Source: three-view drawing plus pictorial views. Frame: mm from the lowest corner of the part. A direction names the side the tool comes from. Round coordinates to 2 decimals unless told otherwise and drop trailing zeros. Loops run counter-clockwise (first coordinate to the right, second up) from the corner with the lowest first, then second, coordinate; pieces in that order, holes last. Notation, with made-up numbers: M 42.5,76.5 L 91.5,76.5 A17 ccw 91.5,98.5 Z; hole C 11,51 d7. An arc over 180 degrees is marked long. Write each question's results on one line, items separated by ' | '.
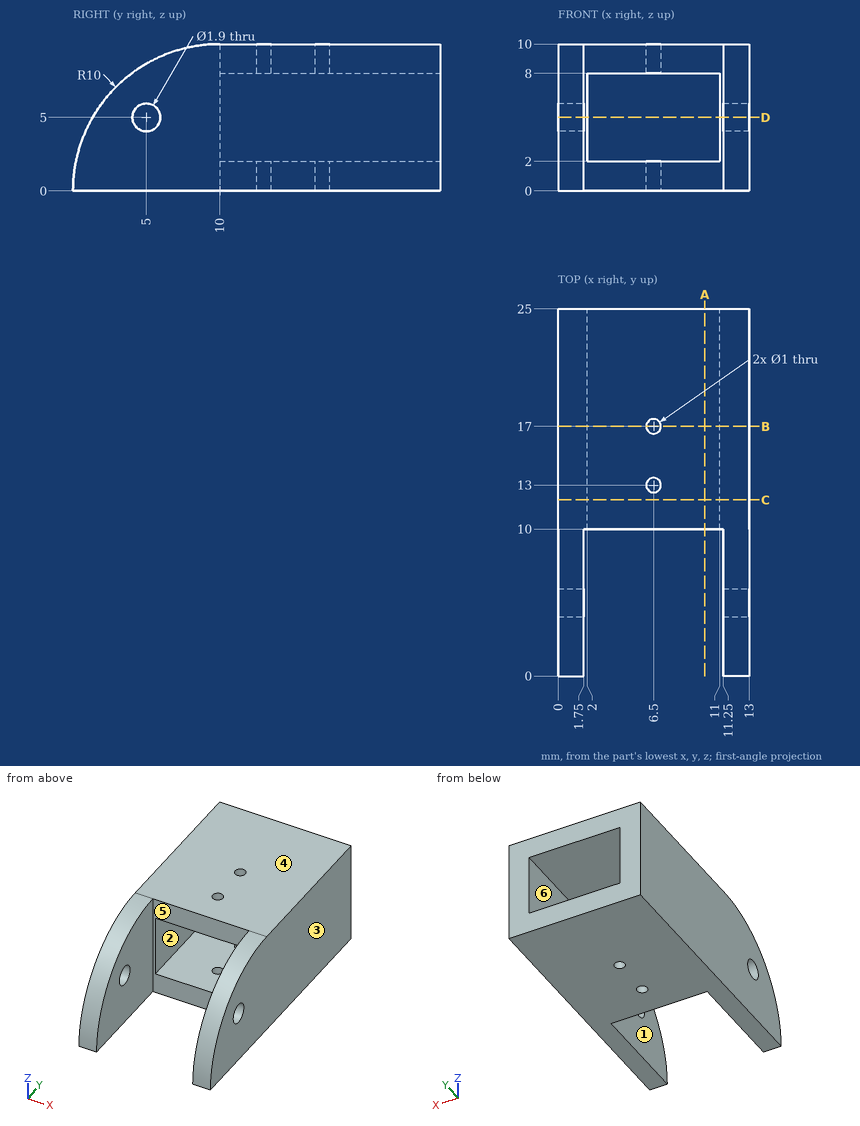
1. Draft query along Z for the marked faces 4, 5 and 6. Return one class per face: pulls with the +Z half, pulls with the -Z half, needs draft (parallel to the pull), parting line crosses it, or undercut.
Answer key:
face 4: pulls with the +Z half | face 5: needs draft | face 6: undercut
2. Section D-D (z = 5). Output: boundary loops of the cut face in (x, y).
Answer key:
outline: M 0,1.34 L 1.75,1.34 L 1.75,4.05 L 0,4.05 Z; M 0,5.95 L 1.75,5.95 L 1.75,10 L 2,10 L 2,25 L 0,25 Z; M 11,10 L 11.25,10 L 11.25,5.95 L 13,5.95 L 13,25 L 11,25 Z; M 11.25,1.34 L 13,1.34 L 13,4.05 L 11.25,4.05 Z
3. Section B-B (y = 17). Output: boundary loops of the cut face in (x, z), then the cut area to 3 significant figures.
Answer key:
outline: M 0,0 L 6,0 L 6,2 L 2,2 L 2,8 L 6,8 L 6,10 L 0,10 Z; M 7,0 L 13,0 L 13,10 L 7,10 L 7,8 L 11,8 L 11,2 L 7,2 Z | area: 72.0 mm²
4. Ray query, probe 1 along Y at (x, z) = (6.5, 0.6); probe 2 along Z at (x, y) = (4.5, 15.25); probe 3 along X at (y, z) = (12.5, 3). Return the intervals inside material, ascending.
Answer key:
probe 1: y = 10 to 12.5, 13.5 to 16.5, 17.5 to 25 | probe 2: z = 0 to 2, 8 to 10 | probe 3: x = 0 to 2, 11 to 13
5. Section C-C (y = 12). Output: boundary loops of the cut face in (x, z), then the cut area to 3 significant figures.
Answer key:
outline: M 0,0 L 13,0 L 13,10 L 0,10 Z; hole M 2,2 L 11,2 L 11,8 L 2,8 Z | area: 76.0 mm²
6. Pin query (flat end, axial travel): P1, Ø6, axis at x = 3, y = 3, coming from the +Z side; P2, Ø5, axis at x = 6.5, z = 6, coming from the -Y side. Return the tip coordinate at first contact, or that it passes through.
Answer key:
P1: stops at z = 9.04 | P2: stops at y = 10
7. Section A-A (x = 10). Output: boundary loops of the cut face in (y, z), then the cut area to 3 significant figures.
Answer key:
outline: M 10,0 L 25,0 L 25,2 L 10,2 Z; M 10,8 L 25,8 L 25,10 L 10,10 Z | area: 60.0 mm²
8. Access query for the marked faces 1, 2 and 3. Directions: +Z, -Z, +X, -X, +Y, -Y. A direction counts if a zero-diameter tool reaches every point of the face in a straight line with its end or side. Return the directions, or none.
Answer key:
face 1: +Z, -Z, -Y | face 2: +Y, -Y | face 3: +Z, -Z, +X, +Y, -Y
